Study the drawing (mm; zero at the part's minimum x, y, z) and answer. A direction names the side the tool comes from. Coordinates: 2 decimals unless noted, no trailing zeros. Loops run counter-clockwise (first coordinate to the right, second up) from the corner with the lowest first, then second, coordinate; pieces in that order, holes last. Notation, with made-up numbers: (26, -33.75) - (79, -33.75) arc R7 cw to (79, -24.75) - close; hole circle Ø8 at (19.5, 44). An arc over 180 degrees is marked (long way). Use one line per item in the form item = value.
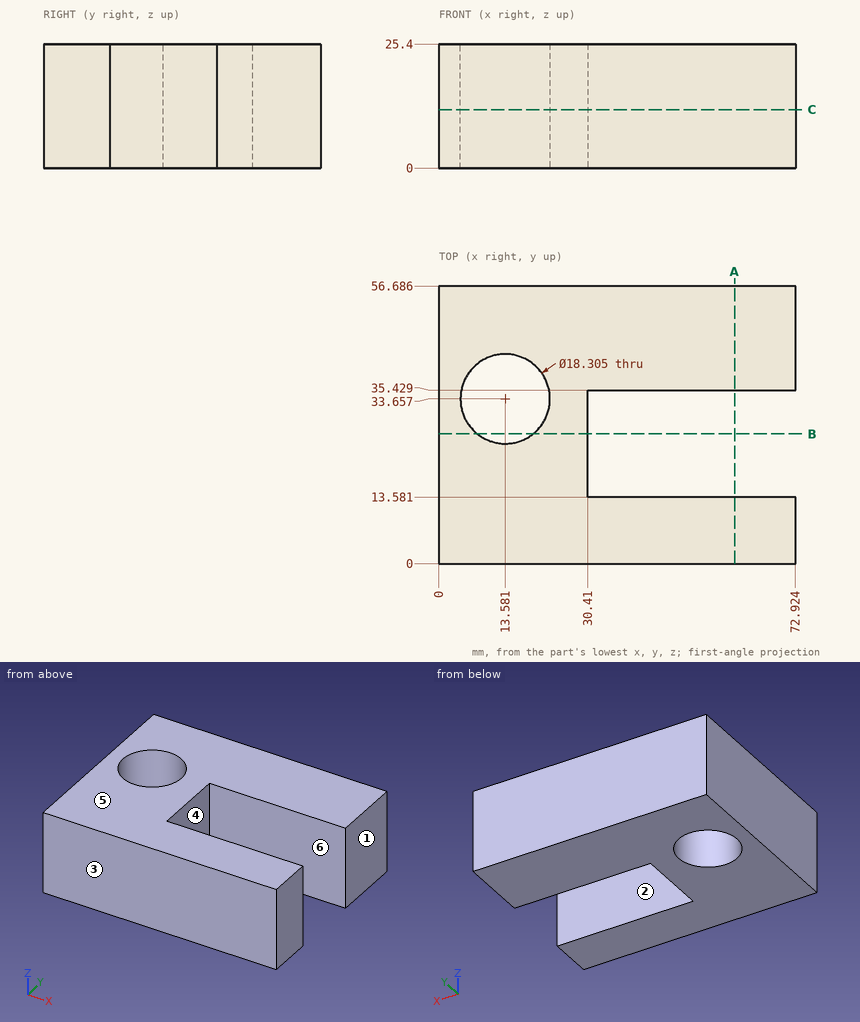
Item 1: The part is cut by section C-C on z = 12. Give the vertices of the cut face in (x, y) (1 decimal).
Results below:
outline = (0, 0) - (72.9, 0) - (72.9, 13.6) - (30.4, 13.6) - (30.4, 35.4) - (72.9, 35.4) - (72.9, 56.7) - (0, 56.7) - close; hole circle Ø18.3 at (13.6, 33.7)
Item 2: For a pull along Y with two mould halves and no side action, classify the marked faces 1, 2, 3 and 4 as +Y half, -Y half, draft (parallel to the pull), parting line (faces both ways), or undercut.
Results below:
face_1 = draft
face_2 = undercut
face_3 = -Y half
face_4 = undercut
Item 3: Find the intervals of material crossed by L1, parallel to Y at x = 56.5, z = 16; L2, parallel to X at y = 17.5, z = 22.5; L3, parallel to X at y = 25.5, z = 4.5, in increasing order.
Results below:
L1 = 0 to 13.58, 35.43 to 56.69
L2 = 0 to 30.41
L3 = 0 to 9.43, 17.73 to 30.41
Item 4: The part is cut by section B-B on y = 26.5. Give the vertices of the cut face in (x, z) (1 decimal), plus the area to 3 significant figures.
Results below:
outline = (0, 0) - (7.9, 0) - (7.9, 25.4) - (0, 25.4) - close; (19.3, 0) - (30.4, 0) - (30.4, 25.4) - (19.3, 25.4) - close
area = 483 mm²
Item 5: Which of the six approach directions +Z, -Z, +X, -X, +Y, -Y give full straight-line access (tool end or side, diameter ignored) to the marked faces 5 and 6?
Results below:
face_5 = +Z, +X, -X, +Y, -Y
face_6 = +Z, -Z, +X
Item 6: The part is cut by section A-A on x = 60.5. Give the vertices of the cut face in (y, z), plus the area to 3 significant figures.
Results below:
outline = (0, 0) - (13.58, 0) - (13.58, 25.4) - (0, 25.4) - close; (35.43, 0) - (56.69, 0) - (56.69, 25.4) - (35.43, 25.4) - close
area = 885 mm²
Item 7: Each of these flat-tipped pins is pushed along its axis until it touches: P1, Ø4, axis at x = 49.5, y = 33, coming from the -Z side; P2, Ø1, axis at x = 37.5, z = 9.5, coming from the -Y side. Where does it stop, or does it pass through?
Results below:
P1 = through
P2 = 0
